from build123d import *

# Parameters (mm, degrees)
SKETCH1_W           = 142.4
SKETCH1_H           = 173.6
BOSS_EXTRUDE1_DEPTH = 4.4
SKETCH2_W           = 142.4
SKETCH2_H           = 5.6
CUT_EXTRUDE1_DEPTH  = 3.2
CUT_EXTRUDE2_REACH  = 114.352
SKETCH3_R           = 1.1
SKETCH4_R           = 0.9
CUT_EXTRUDE3_DEPTH  = 9
CHAMFER2_SIZE       = 0.9
BOSS_EXTRUDE2_DEPTH = 3.2
SKETCH6_R           = 1.1
CUT_EXTRUDE4_DEPTH  = 118.047682591
CUT_EXTRUDE5_DEPTH  = 1.8
CUT_EXTRUDE6_DEPTH  = 0.4


with BuildPart() as part:
    # Sketch1 → Boss-Extrude1 (new body)
    with BuildSketch(Plane(origin=(0, 0, 0), x_dir=(1, 0, 0), z_dir=(0, 1, 0))):
        Rectangle(SKETCH1_W, SKETCH1_H)
    extrude(amount=-BOSS_EXTRUDE1_DEPTH)

    # Sketch2 → Cut-Extrude1 (cut)
    with BuildSketch(Plane.XZ.offset(4.4)):
        with Locations((0, 84)):
            Rectangle(SKETCH2_W, SKETCH2_H)
    extrude(amount=-CUT_EXTRUDE1_DEPTH, mode=Mode.SUBTRACT)

    # Sketch3 → Cut-Extrude2 (cut, up to next)
    with BuildSketch(Plane(origin=(0, 0, 0), x_dir=(1, 0, 0), z_dir=(0, 1, 0)), mode=Mode.PRIVATE) as cut_extrude2_sk1:
        with Locations(Location((60, -84.2, 0), (0, 0, 270))):
            Circle(SKETCH3_R)
    cut_extrude2_tool1 = extrude(cut_extrude2_sk1.sketch, amount=-CUT_EXTRUDE2_REACH, mode=Mode.PRIVATE) & part.part
    # Sketch3 → Cut-Extrude2 (cut, up to next)
    with BuildSketch(Plane(origin=(0, 0, 0), x_dir=(1, 0, 0), z_dir=(0, 1, 0)), mode=Mode.PRIVATE) as cut_extrude2_sk2:
        with Locations(Location((-60, -84.2, 0), (0, 0, 270))):
            Circle(SKETCH3_R)
    cut_extrude2_tool2 = extrude(cut_extrude2_sk2.sketch, amount=-CUT_EXTRUDE2_REACH, mode=Mode.PRIVATE) & part.part
    # Sketch3 → Cut-Extrude2 (cut, up to next)
    with BuildSketch(Plane(origin=(0, 0, 0), x_dir=(1, 0, 0), z_dir=(0, 1, 0)), mode=Mode.PRIVATE) as cut_extrude2_sk3:
        with Locations(Location((0, -84.2, 0), (0, 0, 270))):
            Circle(SKETCH3_R)
    cut_extrude2_tool3 = extrude(cut_extrude2_sk3.sketch, amount=-CUT_EXTRUDE2_REACH, mode=Mode.PRIVATE) & part.part
    add(cut_extrude2_tool1.solids().sort_by_distance((60, 0, 84.2))[0], mode=Mode.SUBTRACT)
    add(cut_extrude2_tool2.solids().sort_by_distance((-60, 0, 84.2))[0], mode=Mode.SUBTRACT)
    add(cut_extrude2_tool3.solids().sort_by_distance((0, 0, 84.2))[0], mode=Mode.SUBTRACT)

    # Sketch4 → Cut-Extrude3 (cut)
    with BuildSketch(Plane(origin=(0, 0, -86.8), x_dir=(-1, 0, 0), z_dir=(0, 0, -1))):
        with Locations((0, -2.2)):
            Circle(SKETCH4_R)
        with Locations((60, -2.2)):
            Circle(SKETCH4_R)
        with Locations((-60, -2.2)):
            Circle(SKETCH4_R)
    extrude(amount=-CUT_EXTRUDE3_DEPTH, mode=Mode.SUBTRACT)

    # Chamfer2
    chamfer2_edges = [part.edges().sort_by_distance(p)[0] for p in [
        (60, 0, 83.1),
        (-60, 0, 83.1),
        (0, 0, 83.1),
    ]]
    chamfer(chamfer2_edges, length=CHAMFER2_SIZE)

    # Sketch5 → Boss-Extrude2 (add)
    with BuildSketch(Plane.XZ.offset(4.4)):
        Polygon((-71.2, 69.858578644), (-78.4, 62.658578644), (-78.4, -62.658578644), (-71.2, -69.858578644), align=None)
        Polygon((71.2, 69.858578644), (78.4, 62.658578644), (78.4, -62.658578644), (71.2, -69.858578644), align=None)
    extrude(amount=-BOSS_EXTRUDE2_DEPTH)

    # Sketch6 → Cut-Extrude4 (cut, through all)
    with BuildSketch(Plane.XZ.offset(4.4)):
        with Locations(Location((74.8, 50, 0), (0, 0, 270))):
            Circle(SKETCH6_R)
        with Locations(Location((74.8, 0, 0), (0, 0, 270))):
            Circle(SKETCH6_R)
        with Locations(Location((74.8, -50, 0), (0, 0, 270))):
            Circle(SKETCH6_R)
        with Locations(Location((-74.8, 50, 0), (0, 0, 270))):
            Circle(SKETCH6_R)
        with Locations(Location((-74.8, 0, 0), (0, 0, 270))):
            Circle(SKETCH6_R)
        with Locations(Location((-74.8, -50, 0), (0, 0, 270))):
            Circle(SKETCH6_R)
    extrude(amount=-CUT_EXTRUDE4_DEPTH, mode=Mode.SUBTRACT)

    # Sketch7 → Cut-Extrude5 (cut)
    with BuildSketch(Plane.XZ.offset(4.4)):
        Polygon((72.4, 48.614359354), (74.8, 47.228718708), (77.2, 48.614359354), (77.2, 51.385640646), (74.8, 52.771281292), (72.4, 51.385640646), align=None)
        Polygon((77.2, 1.385640646), (74.8, 2.771281292), (72.4, 1.385640646), (72.4, -1.385640646), (74.8, -2.771281292), (77.2, -1.385640646), align=None)
        Polygon((77.2, -48.614359354), (74.8, -47.228718708), (72.4, -48.614359354), (72.4, -51.385640646), (74.8, -52.771281292), (77.2, -51.385640646), align=None)
        Polygon((-72.4, -51.385640646), (-72.4, -48.614359354), (-74.8, -47.228718708), (-77.2, -48.614359354), (-77.2, -51.385640646), (-74.8, -52.771281292), align=None)
        Polygon((-72.4, -1.385640646), (-72.4, 1.385640646), (-74.8, 2.771281292), (-77.2, 1.385640646), (-77.2, -1.385640646), (-74.8, -2.771281292), align=None)
        Polygon((-72.4, 48.614359354), (-72.4, 51.385640646), (-74.8, 52.771281292), (-77.2, 51.385640646), (-77.2, 48.614359354), (-74.8, 47.228718708), align=None)
    extrude(amount=-CUT_EXTRUDE5_DEPTH, mode=Mode.SUBTRACT)

    # Sketch8 → Cut-Extrude6 (cut)
    with BuildSketch(Plane.XZ.offset(4.4)):
        Polygon((78.4, -17.9), (-29.05, -17.9), (-44.95, -33.8), (-44.95, -86.8), (-29.05, -86.8), (-29.05, -33.8), (78.4, -33.8), align=None)
    extrude(amount=-CUT_EXTRUDE6_DEPTH, mode=Mode.SUBTRACT)


solid = part.part
Geometry check sheet. Reference: the model listing, model coordinates, mm. A direction names the side the tool comes from. Give positions to 0.01 mm unless a question says otherwise; leave off trailing zeros. Write each loop counter-clockwise with the first axis right and the second up, starting at its lowest first coordinate (ties: lowest second). Pieces come first, ordered by that corner, then holes.
1) Cross-section at D-D (x = -64.5). Record the boundary of the cut face in (y, z).
Values follow:
outline: (-4.4, -86.8) - (0, -86.8) - (0, 86.8) - (-1.2, 86.8) - (-1.2, 81.2) - (-4.4, 81.2) - close
2) Thickness scan on line 1 (X direction, y = -2, z = 50); line 2 (Z direction, x = 17, y = -4.15); line 3 (Y direction, x = -60, z = -80.5). Record the ranges inside material, lowest first.
Values follow:
line 1: x = -78.4 to -75.9, -73.7 to 73.7, 75.9 to 78.4
line 2: z = -86.8 to -33.8, -17.9 to 81.2
line 3: y = -4.4 to -3.1, -1.3 to 0
3) Cross-section at A-A (z = 17). Record the boundary of the cut face in (x, y).
Values follow:
outline: (-78.4, -4.4) - (78.4, -4.4) - (78.4, -1.2) - (71.2, -1.2) - (71.2, 0) - (-71.2, 0) - (-71.2, -1.2) - (-78.4, -1.2) - close
4) Set-up check for faces 4 (the face through (74, -1.2, 1)), 5 (the face through (-76, -2.6, 49)), 6 (the face through (-36.89, -4.2, -25.74)), 7 (the face through (-71.2, -1, 1)): record each of +Z, -Z, +X, -X, +Y, -Y from which the full face is reachable in a straight line by a thin tool's end or side.
Values follow:
face 4: +Z, -Z, +X, +Y
face 5: -Y
face 6: -Z, +X, -Y
face 7: -X, +Y
5) Cross-section at C-C (x = -13.5). Record the boundary of the cut face in (y, z), plus the area to 3 significant figures.
Values follow:
outline: (-4.4, -86.8) - (0, -86.8) - (0, 86.8) - (-1.2, 86.8) - (-1.2, 81.2) - (-4.4, 81.2) - (-4.4, -17.9) - (-4, -17.9) - (-4, -33.8) - (-4.4, -33.8) - close
area: 740 mm2
6) Cross-section at B-B (x = -33.5). Record the boundary of the cut face in (y, z), plus the area to 3 significant figures.
Values follow:
outline: (-4.4, -22.35) - (-4, -22.35) - (-4, -86.8) - (0, -86.8) - (0, 86.8) - (-1.2, 86.8) - (-1.2, 81.2) - (-4.4, 81.2) - close
area: 720 mm2
7) Go/stop test with flat-tipped pins: pin 1 Ø2.5 at (x, z) = (-74, 49.5) entering from -Y; pin 2 Ø1.3 at (x, z) = (-74.8, -50) entering from -Y; pin 3 Ø5.5 at (x, z) = (74, 49) entering from -Y; pin 4 Ø0.5 at (x, y) = (0, -2.5) entering from -Z. Record where each tip stops, or that it passes through.
Values follow:
pin 1: stops at y = -2.6
pin 2: passes through
pin 3: stops at y = -4.4
pin 4: stops at z = -77.8
8) Release check for a two-part mould opening along X. For faces 1 (the face through (71.2, -1, 1)), 2 (the face through (74, -2.6, -51)), 3 (the face through (-19, -4.4, 15)) record: released by +X, released by -X, zero draft, split by the parting line, or undercut.
Values follow:
face 1: released by +X
face 2: undercut
face 3: zero draft
